Can you work these out from the model? Positions are in its coordinate system, mm. A direction names the side the tool comes from. Coordinates: 2 decimals unless noted, no trailing zeros. Order: outer loops, then holes, each group sorted by start corner. A loop starts at its lowest first (then second) coordinate and runs counter-clockwise, first axis right, second up. Notation, with made-up numbers: (0, 79.25) - (11, 79.25) arc R36 cw to (11, 113.25) - close; hole circle Ø7 at (20, 7). An arc over 180 degrees is marked (long way). Use a Markdown table: item, result. Add a question column.
(1) If I drill on L1, parallel to Y at x = 0.5, z = 65.97; L2, parallel to Z at x = -1.25, y = -0.75; L3, parallel to Z at x = 6.5, y = -1, over which ranges is the centre line in solid material (lowest first)? Write a range as [from, to].
(2) I want a section at D-D (z = -34). List the corners of the cut face in (x, y) for me.
(3) I want a section at A-A (z = 65.97). List the corners of the cut face in (x, y) for me.
(4) On a 3-axis mill with a long thin cutter (end or side, diameter ignored), from which of +Z, -Z, +X, -X, +Y, -Y can I reach the whole of each face in a straight line? I mean faces 4 (the flat face through (3.25, -2, -41)), 5 (the flat face through (-4.35, -0.1, 63.9)), 6 (the flat face through (-6.4, 0.1, 0)). Say none if no direction works.
(5) For pin 1 Ø3 at (y, z) = (0, 65.5) entering from +X; pin 2 Ø9.5 at (y, z) = (3, -20.5) entering from +X; pin 3 Ø5 at (y, z) = (0, -44) entering from -X; pin 4 Ø2.5 at (y, z) = (0, -42.4) entering from +X, each with a flat end and sliding along its axis, tell me the tip position at first contact or that it passes through.
(6) I want a section at C-C (x = 7.5). List the corners of the cut face in (y, z) for me, and give its area (3 significant figures).
(7) We'd pull the mould along Z, two halves only. Please class faces 1 (the flat face through (0, 0, -46.4)), 2 (the flat face through (-8.364, -10.244, 30.246)), 3 (the cylindrical face through (0.046, 0.616, -44.355)): pulls with the +Z half, pulls with the -Z half, needs draft (parallel to the pull), parting line crosses it, or undercut.
(8) I want a section at B-B (x = 0). List the corners of the cut face in (y, z) for me.
```python
from build123d import *
from OCP.BRepFilletAPI import BRepFilletAPI_MakeChamfer

# Parameters (mm, degrees)
SKETCH1_W           = 18.7
SKETCH1_H           = 24
BOSS_EXTRUDE1_DEPTH = 61.35
CHAMFER1_SIZE       = 2
CHAMFER1_SIZE2      = 3.464101615
CHAMFER2_SIZE       = 2
CHAMFER3_SIZE       = 2
CHAMFER3_SIZE2      = 11.342563639
SKETCH2_W           = 12
SKETCH2_H           = 12
BOSS_EXTRUDE2_DEPTH = 35.4
SKETCH3_R           = 4.5
BOSS_EXTRUDE3_DEPTH = 11
CUT_EXTRUDE1_START  = -8
CUT_EXTRUDE1_DEPTH  = 8
SKETCH5_W           = 8.5
SKETCH5_H           = 10
BOSS_EXTRUDE4_DEPTH = 9.24
SKETCH7_R           = 1.9
CUT_EXTRUDE2_DEPTH  = 10
FILLET1_R           = 1.5
SKETCH8_R           = 2.05
CUT_EXTRUDE3_DEPTH  = 73.702875459


with BuildPart() as part:
    # Sketch1 → Boss-Extrude1 (new body)
    with BuildSketch(Plane.XY):
        Rectangle(SKETCH1_W, SKETCH1_H)
    extrude(amount=BOSS_EXTRUDE1_DEPTH)

    # Chamfer1: one chamfer whose edges measure the first distance from different faces: ONE call of the kernel's chamfer builder (chamfer() names one face for all edges)
    chamfer1_edges_1 = [part.edges().sort_by_distance(p)[0] for p in [
        (-9.35, 12, 30.675),
    ]]
    chamfer1_side_1 = [part.faces().sort_by_distance(p)[0] for p in [
        (0, 12, 30.675),
    ]]
    chamfer1_edges_2 = [part.edges().sort_by_distance(p)[0] for p in [
        (-9.35, -12, 30.675),
    ]]
    chamfer1_side_2 = [part.faces().sort_by_distance(p)[0] for p in [
        (0, -12, 30.675),
    ]]
    chamfer1 = BRepFilletAPI_MakeChamfer(part.part.solid().wrapped)
    for e in chamfer1_edges_1:
        chamfer1.Add(CHAMFER1_SIZE, CHAMFER1_SIZE2, e.wrapped, chamfer1_side_1[0].wrapped)  # the first distance lies on this face
    for e in chamfer1_edges_2:
        chamfer1.Add(CHAMFER1_SIZE, CHAMFER1_SIZE2, e.wrapped, chamfer1_side_2[0].wrapped)  # the first distance lies on this face
    add(Compound.cast(chamfer1.Shape()), mode=Mode.REPLACE)

    # Chamfer2
    chamfer2_edges = [part.edges().sort_by_distance(p)[0] for p in [
        (1, -12, 0),
        (1, 12, 61.35),
        (1, -12, 61.35),
    ]]
    chamfer(chamfer2_edges, length=CHAMFER2_SIZE)

    # Chamfer3
    chamfer3_edges = [part.edges().sort_by_distance(p)[0] for p in [
        (1, 12, 0),
    ]]
    chamfer3_side = [part.faces().sort_by_distance(p)[0] for p in [
        (0.087625567, 0.932238812, 0),
    ]]
    chamfer(chamfer3_edges, length=CHAMFER3_SIZE, length2=CHAMFER3_SIZE2, reference=chamfer3_side[0])

    # Sketch2 → Boss-Extrude2 (add)
    with BuildSketch(Plane(origin=(0, 0, 0), x_dir=(-1, 0, 0), z_dir=(0, 0, -1))):
        Rectangle(SKETCH2_W, SKETCH2_H)
    extrude(amount=BOSS_EXTRUDE2_DEPTH)

    # Sketch3 → Boss-Extrude3 (add)
    with BuildSketch(Plane(origin=(0, 0, -35.4), x_dir=(-1, 0, 0), z_dir=(0, 0, -1))):
        Circle(SKETCH3_R)
    extrude(amount=BOSS_EXTRUDE3_DEPTH)

    # Sketch4 → Cut-Extrude1 (cut)
    with BuildSketch(Plane(origin=(0, 0, -46.4), x_dir=(-1, 0, 0), z_dir=(0, 0, -1)).offset(CUT_EXTRUDE1_START)):
        with BuildLine():
            ThreePointArc((-3.25, 3.112474899), (-4.5, 0), (-3.25, -3.112474899))
            Line((-3.25, -3.112474899), (-3.25, 3.112474899))
        make_face()
        with BuildLine():
            Line((3.25, 3.112474899), (3.25, -3.112474899))
            ThreePointArc((3.25, -3.112474899), (4.175823272, -1.677050983), (4.5, 0))
            ThreePointArc((4.5, 0), (4.175823272, 1.677050983), (3.25, 3.112474899))
        make_face()
    extrude(amount=CUT_EXTRUDE1_DEPTH, mode=Mode.SUBTRACT)

    # Sketch5 → Boss-Extrude4 (add)
    with BuildSketch(Plane.XY.offset(61.35)):
        with Locations((-0.1, 0)):
            Rectangle(SKETCH5_W, SKETCH5_H)
    extrude(amount=BOSS_EXTRUDE4_DEPTH)

    # Sketch7 → Cut-Extrude2 (cut)
    with BuildSketch(Plane(origin=(4.15, 0, 0), x_dir=(0, 0, -1), z_dir=(1, 0, 0))):
        with Locations((-65.97, 0)):
            Circle(SKETCH7_R)
    extrude(amount=-CUT_EXTRUDE2_DEPTH, mode=Mode.SUBTRACT)

    # Fillet1
    fillet1_edges = [part.edges().sort_by_distance(p)[0] for p in [
        (-0.1, 5, 70.59),
        (-0.1, -5, 70.59),
    ]]
    fillet(fillet1_edges, radius=FILLET1_R)

    # Sketch8 → Cut-Extrude3 (cut, through all)
    with BuildSketch(Plane(origin=(3.25, 0, 0), x_dir=(0, 0, -1), z_dir=(1, 0, 0))):
        with Locations((42.4, 0)):
            Circle(SKETCH8_R)
    extrude(amount=-CUT_EXTRUDE3_DEPTH, mode=Mode.SUBTRACT)


solid = part.part
```
Answers follow:
| question | item | result |
|---|---|---|
| 1 | L1 | y = [-5, -1.9], [1.9, 5] |
| 1 | L2 | z = [-46.4, -44.31], [-40.49, 64.22], [67.72, 70.59] |
| 1 | L3 | z = [0, 61.35] |
| 2 | outline | (-6, -6) - (6, -6) - (6, 6) - (-6, 6) - close |
| 3 | outline | (-4.35, -5) - (4.15, -5) - (4.15, -1.9) - (-4.35, -1.9) - close; (-4.35, 1.9) - (4.15, 1.9) - (4.15, 5) - (-4.35, 5) - close |
| 4 | face 4 | -Z, +X, +Y, -Y |
| 4 | face 5 | +Z, -X, +Y, -Y |
| 4 | face 6 | -Z |
| 5 | pin 1 | stops at x = 4.15 |
| 5 | pin 2 | stops at x = 6 |
| 5 | pin 3 | stops at x = -3.25 |
| 5 | pin 4 | passes through |
| 6 | outline | (-12, 2) - (-10, 0) - (10, 0) - (12, 11.34) - (12, 59.35) - (10, 61.35) - (-10, 61.35) - (-12, 59.35) - close |
| 6 | area | 1,460 mm² |
| 7 | face 1 | pulls with the -Z half |
| 7 | face 2 | needs draft |
| 7 | face 3 | undercut |
| 8 | outline | (-12, 2) - (-10, 0) - (-6, 0) - (-6, -35.4) - (-4.5, -35.4) - (-4.5, -46.4) - (4.5, -46.4) - (4.5, -35.4) - (6, -35.4) - (6, 0) - (10, 0) - (12, 11.34) - (12, 59.35) - (10, 61.35) - (5, 61.35) - (5, 69.09) arc R1.5 ccw to (3.5, 70.59) - (-3.5, 70.59) arc R1.5 ccw to (-5, 69.09) - (-5, 61.35) - (-10, 61.35) - (-12, 59.35) - close; hole circle Ø4.1 at (0, -42.4); hole circle Ø3.8 at (0, 65.97) |
